Design review of the part shown in the three views and the two pictorial views. Dimensions are in mm from the part's minimum x, y and z. Give positions to 0.01 mm unless a question says otherwise; leave off trailing zeros. Write each loop counter-clockwise with the first axis right and the second up, starting at its lowest first coordinate (ties: lowest second). Pieces come first, ordered by that corner, then holes. Notation, with made-up numbers: M -5,62.5 L 3,62.5 A25 ccw 3,92.5 Z; hole C -7,53 d8. An arc over 180 degrees is marked long. Use one line per item in the form item = value. Start each with the question number.
Q1. For probe 1 along Z at (x, y) = (506.5, 87); probe 2 along Z at (x, y) = (1316.5, 302.5), list the stretches that pass through material, from the lowest coordinate up. Write a range as [from, to].
Q2. Consider section A-A on x = 1326. Write out the cut boundary in (y, z), and give its area (3 significant figures).
Q3. Consider section C-C on y = 136. Write out the cut boundary in (x, z) (3 decimals), and give its area (3 significant figures).
Q4. Clearance check with flat-ended pins moving along their axes: pin 1 Ø7.5 at (x, z) = (1908, 376) entering from -Y; pin 2 Ø20.5 at (y, z) = (291.5, 349.5) entering from +X (3 decimals); pin 3 Ø20.5 at (y, z) = (289.5, 341) entering from -X (3 decimals). State where each tip first meets the part, or that it passes through.
Q5. Consider section B-B on z = 620. Write out the cut boundary in (x, y) (3 decimals).
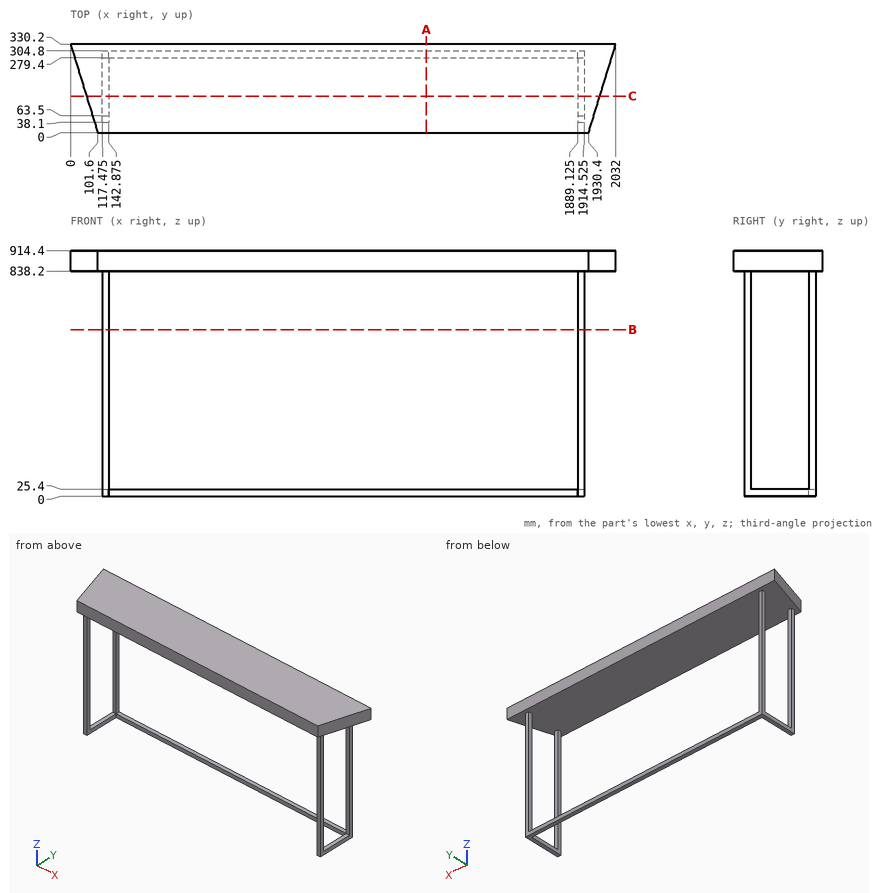
Working result:
q1.probe_1 = [838.2, 914.4]
q1.probe_2 = [0, 25.4], [838.2, 914.4]
q2.outline = M 0,838.2 L 330.2,838.2 L 330.2,914.4 L 0,914.4 Z; M 279.4,0 L 304.8,0 L 304.8,25.4 L 279.4,25.4 Z
q2.area = 25,800 mm²
q3.outline = M 59.754,838.2 L 1972.246,838.2 L 1972.246,914.4 L 59.754,914.4 Z; M 117.475,0 L 142.875,0 L 142.875,25.4 L 117.475,25.4 Z; M 1889.125,0 L 1914.525,0 L 1914.525,25.4 L 1889.125,25.4 Z
q3.area = 147,000 mm²
q4.pin_1 = 38.1
q4.pin_2 = 1914.525
q4.pin_3 = 117.475
q5.outline = M 117.475,38.1 L 142.875,38.1 L 142.875,63.5 L 117.475,63.5 Z; M 117.475,279.4 L 142.875,279.4 L 142.875,304.8 L 117.475,304.8 Z; M 1889.125,38.1 L 1914.525,38.1 L 1914.525,63.5 L 1889.125,63.5 Z; M 1889.125,279.4 L 1914.525,279.4 L 1914.525,304.8 L 1889.125,304.8 Z
